Read the model definition and answer for the solid it produces. Units are mm, in the model's axes. A direction names the side the tool comes from. Coordinates: 2 decimals unless noted, no trailing zeros. Loops run counter-clockwise (first coordinate to the right, second up) from the corner with the lowest first, then second, coordinate; pieces in that order, holes last. Notation, with made-up numbers: (44, 70) -> (55, 70) arc R14 cw to (55, 80) -> close; hole circle Ø2 at (64, 11). An arc over 180 degrees is marked (long way). Answer as CSV lines item,"result".
```python
from build123d import *

# Parameters (mm, degrees)
F2_W     = 127
F2_H     = 162.576706
F3_DEPTH = 12.7
F4_W     = 105.833333
F4_H     = 120.243372
F5_DEPTH = 12.7
F6_DEPTH = 254
F1_W     = 66.04
F1_H     = 177.8
F7_DEPTH = 7.62


with BuildPart() as f3:
    # F2 (on Top) → F3 (new body)
    with BuildSketch(Plane.XY):
        with Locations((63.5, 366.946444)):
            Rectangle(F2_W, F2_H)
    extrude(amount=F3_DEPTH)

    # F4 (on face) → F5 (join)
    with BuildSketch(Plane.XY.offset(12.7)):
        with Locations((52.916666, 366.946444)):
            Rectangle(F4_W, F4_H)
    extrude(amount=F5_DEPTH)

    # F0 (on Right) → F6 (join)
    with BuildSketch(Plane.YZ):
        Polygon((0, 228.6), (0, 0), (508, 0), (508, 228.6), (254, 304.8), align=None)
    extrude(amount=-F6_DEPTH)

    # F1 (on Right) → F7 (cut)
    with BuildSketch(Plane.YZ):
        with Locations((373.38, 114.3)):
            Rectangle(F1_W, F1_H)
    extrude(amount=-F7_DEPTH, mode=Mode.SUBTRACT)


solid = f3.part
```
Q1. For a pull along Y with two mould halves and no side action, classify faces 1 (the face through (-7.62, 373, 116)), 2 (the face through (63, 285.658, 6)), 3 (the face through (105.833, 366, 19)), 4 (the face through (-125, 508, 113)) as pulls with the +Y half, pulls with the -Y half, needs draft (parallel to the pull), parting line crosses it, or undercut.
Results:
face 1,"undercut"
face 2,"pulls with the -Y half"
face 3,"needs draft"
face 4,"pulls with the +Y half"
Q2. Find the intervals of material crossed by probe 1 along X at (y, z) = (129, 147); probe 2 along Z at (x, y) = (45.5, 333.5); probe 3 along X at (y, z) = (413, 20), in increasing order. Write a range as [from, to].
Results:
probe 1,"x = [-254, 0]"
probe 2,"z = [0, 25.4]"
probe 3,"x = [-254, 105.83]"
Q3. For faces 5 (the face through (52, 306.825, 19)), 6 (the face through (52, 427.068, 19)), 7 (the face through (63, 448.235, 6)), determine the directions among +Z, -Z, +X, -X, +Y, -Y from which every point of the face is accessible in a straight line to the end or side of a thin tool.
Results:
face 5,"+Z, +X, -Y"
face 6,"+Z, +X, +Y"
face 7,"+Z, -Z, +X, +Y"
Q4. A cutting plane is placed at D-D, the plane x = -38.5. Write down the section's boundary in (y, z), and give its area (3 significant figures).
Results:
outline,"(0, 0) -> (508, 0) -> (508, 228.6) -> (254, 304.8) -> (0, 228.6) -> close"
area,"135,000 mm²"
Q5. Given pin 1 Ø6 at (y, z) = (305.5, 87.5) entering from +X; pin 2 Ø10 at (x, z) = (92.5, 7) entering from -Y; pin 3 Ø10 at (x, z) = (71.5, 8.5) entering from +Y, each flat-ended and moving along its own axis, determine where each tip first touches the part or whether it passes through.
Results:
pin 1,"stops at x = 0"
pin 2,"stops at y = 285.66"
pin 3,"stops at y = 448.23"
Q6. A cutting plane is placed at B-B, the plane z = 170.5. Write down the section's boundary in (x, y).
Results:
outline,"(-254, 0) -> (0, 0) -> (0, 340.36) -> (-7.62, 340.36) -> (-7.62, 406.4) -> (0, 406.4) -> (0, 508) -> (-254, 508) -> close"
Q7. A cutting plane is placed at C-C, the plane x = 45. Write down the section's boundary in (y, z).
Results:
outline,"(285.66, 0) -> (448.23, 0) -> (448.23, 12.7) -> (427.07, 12.7) -> (427.07, 25.4) -> (306.82, 25.4) -> (306.82, 12.7) -> (285.66, 12.7) -> close"
Q8. A cutting plane is placed at A-A, the plane y = 438.5. Write down the section's boundary in (x, z).
Results:
outline,"(-254, 0) -> (127, 0) -> (127, 12.7) -> (0, 12.7) -> (0, 249.45) -> (-254, 249.45) -> close"
